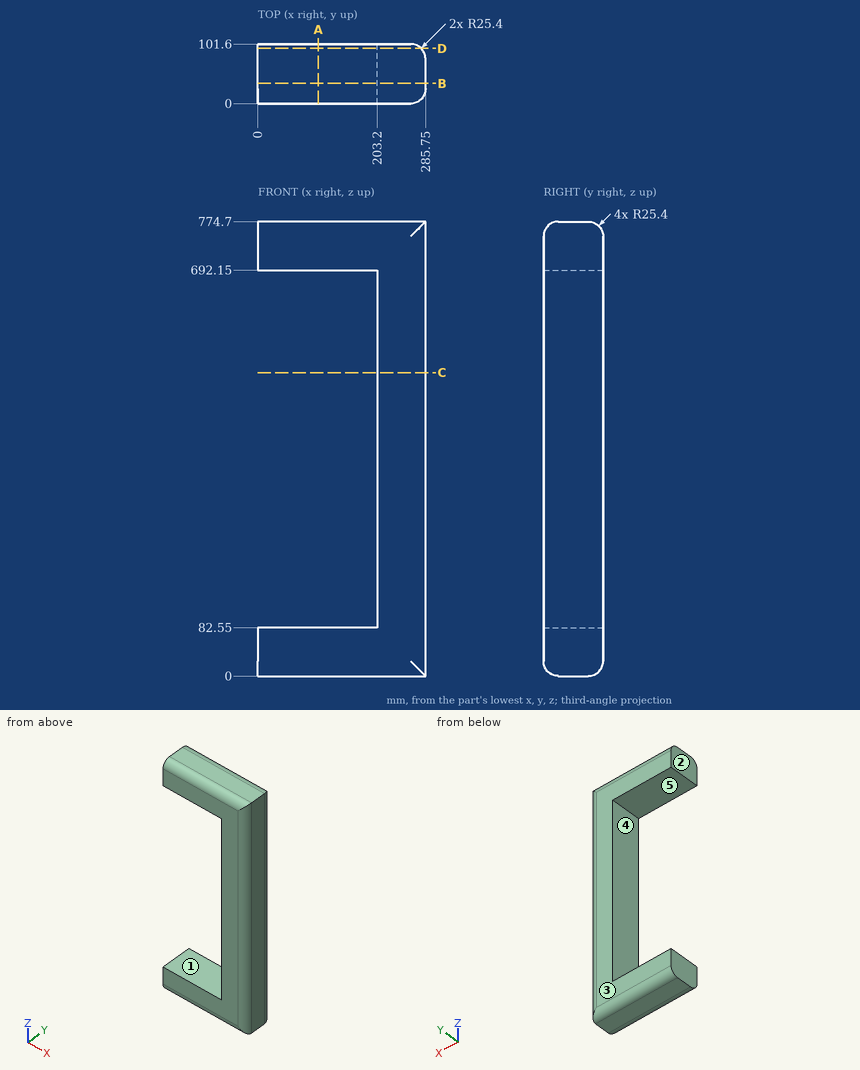
Drawing for the job (mm, zero at the part's lowest x, y, z). A direction names the side the tool comes from. Coordinates: 2 decimals unless noted, no trailing zeros. Loops run counter-clockwise (first coordinate to the right, second up) from the corner with the lowest first, then second, coordinate; pieces in that order, holes last. Notation, with made-up numbers: (53, -16.5) - (84, -16.5) arc R16 cw to (84, 0.5) - close; hole circle Ø5 at (-28, -35). An arc over 180 degrees is marked (long way). Use CSV: the item, a comma, the result in double quotes. Start each with the question number.
Q1. Probe probe 1 along Z at (x, y) = (142, 30); probe 2 along X at (y, z) = (71, 368.5); probe 3 along Z at (x, y) = (195, 91.5). List the from-to ranges inside material, lowest first. Write a range as from..to.
Q2. Cut at C-C, the plane z = 517. List the corners of the cut face in (x, y), then the cut area to 3 significant figures.
Q3. Cut at D-D, the plane y = 94. List the corners of the cut face in (x, z), then the cut area to 3 significant figures.
Q4. 3-axis set-ups, long thin cutter, end or side, ignore diameter. For the marked faces 1 and 2: which of +Z, -Z, +X, -X, +Y, -Y reach the whole face in a straight line?
Q5. Cut at A-A, the plane x = 103. List the corners of the cut face in (y, z), then the cut area to 3 significant figures.
Q6. Two-plate mould, pull along Z, no slides. Class the marked faces 3, 4 and 5: +Z half, -Z half, draft (parallel to the pull), parting line (faces both ways), or undercut.
Q7. Drop flat-ended pins along their axis: P1, Ø1.5, axis at x = 245, y = 83.5, coming from the -Z side; P2, Ø5, axis at y = 76.5, z = 528.5, coming from the -X side; P3, Ø6, axis at x = 118, y = 13.5, coming from the +Z side. Give the stop position or say it passes through.
Q8. Cut at B-B, the plane y = 34.5. List the corners of the cut face in (x, z), then the cut area to 3 significant figures.
Here are the results:
1,probe 1,"0..82.55, 692.15..774.7"
1,probe 2,"203.2..285.75"
1,probe 3,"5.13..82.55, 692.15..769.57"
2,outline,"(203.2, 0) - (260.35, 0) arc R25.4 ccw to (285.75, 25.4) - (285.75, 76.2) arc R25.4 ccw to (260.35, 101.6) - (203.2, 101.6) - close"
2,area,"8,110 mm2"
3,outline,"(0, 7.28) - (278.47, 7.28) - (278.47, 767.42) - (0, 767.42) - (0, 692.15) - (203.2, 692.15) - (203.2, 82.55) - (0, 82.55) - close"
3,area,"87,800 mm2"
4,face 1,"-X, +Y, -Y"
4,face 2,"+Z, -Z, -X, +Y, -Y"
5,outline,"(0, 25.4) arc R25.4 ccw to (25.4, 0) - (76.2, 0) arc R25.4 ccw to (101.6, 25.4) - (101.6, 82.55) - (0, 82.55) - close; (0, 692.15) - (101.6, 692.15) - (101.6, 749.3) arc R25.4 ccw to (76.2, 774.7) - (25.4, 774.7) arc R25.4 ccw to (0, 749.3) - close"
5,area,"16,200 mm2"
6,face 3,"draft"
6,face 4,"undercut"
6,face 5,"undercut"
7,P1,"z = 0.86"
7,P2,"x = 203.2"
7,P3,"z = 773.09"
8,outline,"(0, 0) - (285.75, 0) - (285.75, 774.7) - (0, 774.7) - (0, 692.15) - (203.2, 692.15) - (203.2, 82.55) - (0, 82.55) - close"
8,area,"97,500 mm2"
